Autodesk Inventor part; units mm, degrees
ref_plane "YZ Plane" through (0, 0, 0) normal (1, 0, 0) x (0, 1, 0)
ref_plane "XZ Plane" through (0, 0, 0) normal (0, 1, 0) x (-1, 0, 0)
ref_plane "XY Plane" through (0, 0, 0) normal (0, 0, 1) x (1, 0, 0)
sketch "Sketch1" plane through (0, 0, 0) normal (0, 0, 1) x (1, 0, 0)
  line L0 (0.35, 0) -> (0.35, 7)
  line L1 (0.35, 7) -> (2.8418, 7)
  arc A0 (4, 5.8) -> (2.8418, 7) centre (2.8418, 5.8411) ccw
  line L2 (4, 5.8) -> (4, 5.5)
  line L3 (4, 5.5) -> (2, 5.5)
  line L4 (2, 5.5) -> (2, 0)
  line L5 (2, 0) -> (0.35, 0)
  line L6 (0, 0) -> (0, 7) construction
  dimension "d0" = 4
  dimension "d1" = 0.7
  dimension "d2" = 7
  dimension "d3" = 1.5
  dimension "d4" = 8
  dimension "d5" = 0.3
revolve "Revolution1" add sketch "Sketch1" angle 360 about axis through (0, 0, 0) along (0, 1, 0)
properties part number "remache"
The model under review builds one solid part; all positions refer to its coordinate system, in mm. A direction names the side the tool comes from. Round coordinates to 2 decimals unless told otherwise and drop trailing zeros. Write each loop counter-clockwise with the first axis right and the second up, starting at its lowest first coordinate (ties: lowest second). Pieces come first, ordered by that corner, then holes. Notation, with made-up numbers: (77, 22) - (110, 22) arc R21 cw to (110, 37) - close; hole circle Ø8 at (73, -5). An arc over 180 degrees is marked (long way). Answer as CSV lines item,"result". Start each with the question number.
(1) For faces 1 (the flat face through (0, 0, -0.5)), 2 (the flat face through (-2, 5.5, 1)), list the 3-axis set-ups (+Z, -Z, +X, -X, +Y, -Y) from which the entire face can be reached by the end or side of a thin tool; tool diameter is ignored.
(2) To check wall thickness, follow line 1 (Z direction, x = 0, y = 2); line 2 (Z direction, x = 0, y = 5.75). State the ranges of each line that lie inside material, in increasing order.
(3) We need section C-C on y = 2. State the section outline as (x, z) points, plus the area to 3 significant figures.
(4) We need section B-B on x = 0. State the section outline as (y, z) points, plus the area to 3 significant figures.
(5) We need section A-A on z = 0. State the section outline as (x, y) points.
(6) For pin 1 Ø3 at (y, z) = (5, -3) entering from +X; pin 2 Ø3 at (x, y) = (0.5, 3) entering from +Z; pin 3 Ø4 at (x, y) = (3, 1) entering from +Z, all flat-tipped, find the tip position at first contact; note any pin that passes through.
Worked answers:
1,face 1,"+Z, -Z, +X, -X, -Y"
1,face 2,"-Y"
2,line 1,"-2 to -0.35, 0.35 to 2"
2,line 2,"-4 to -0.35, 0.35 to 4"
3,outline,"circle Ø4 at (0, 0); hole circle Ø0.7 at (0, 0)"
3,area,"12.2 mm²"
4,outline,"(0, -2) - (5.5, -2) - (5.5, -4) - (5.8, -4) arc R1.16 ccw to (7, -2.84) - (7, -0.35) - (0, -0.35) - close; (0, 0.35) - (7, 0.35) - (7, 2.84) arc R1.16 ccw to (5.8, 4) - (5.5, 4) - (5.5, 2) - (0, 2) - close"
4,area,"28.5 mm²"
5,outline,"(-4, 5.5) - (-2, 5.5) - (-2, 0) - (-0.35, 0) - (-0.35, 7) - (-2.84, 7) arc R1.16 ccw to (-4, 5.8) - close; (0.35, 0) - (2, 0) - (2, 5.5) - (4, 5.5) - (4, 5.8) arc R1.16 ccw to (2.84, 7) - (0.35, 7) - close"
6,pin 1,"x = 3.67"
6,pin 2,"z = 2"
6,pin 3,"z = 1.73"
